Source: three-view drawing plus pictorial views. Frame: mm from the lowest corner of the part. A direction names the side the tool comes from. Coordinates: 2 decimals unless noted, no trailing zeros. Write each loop counter-clockwise with the first axis right and the second up, starting at its lowest first coordinate (ties: lowest second). Pieces come first, ordered by that corner, then holes. Notation, with made-up numbers: (-23.5, 80.25) -> (-3.5, 80.25) arc R23 cw to (-3.5, 94.25) -> close; hole circle Ø2 at (-36, 80.25). An arc over 180 degrees is marked (long way). One line per item, written item: value. Start each with the question number.
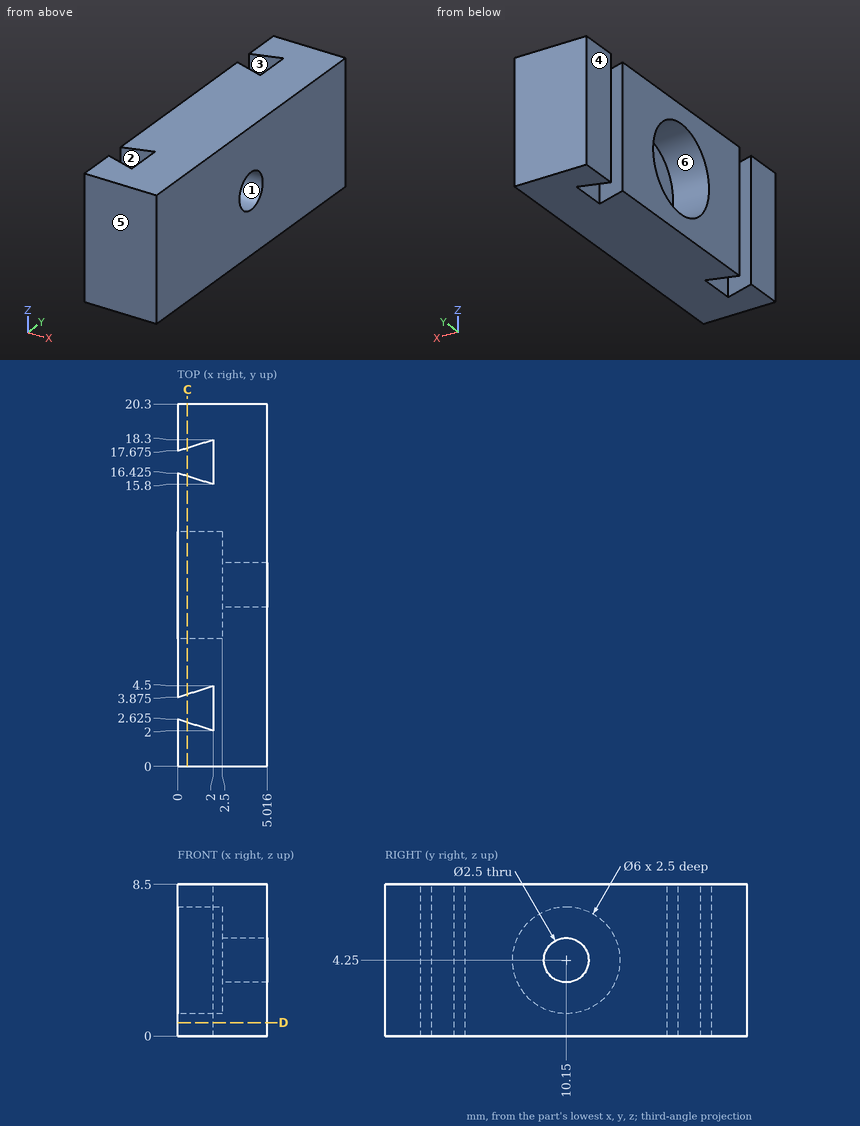
Q1. Draft query along Y for the marked faces 3, 4, 5 and 6. Return one class per face: pulls with the +Y half, pulls with the -Y half, needs draft (parallel to the pull), parting line crosses it, or undercut.
Q2. Access query for the marked faces 1 and 2. Directions: +Z, -Z, +X, -X, +Y, -Y. A direction counts if a zero-diameter tool reaches every point of the face in a straight line with its end or side. Return the directions, or none.
Q3. Line query: L1, parallel to Y at x = 3.5, z = 4.25; L2, parallel to Y at x = 1.8, z = 3; L3, parallel to Y at x = 0.9, z = 3.5 (1 decimal). Output: solid intervals per line, ascending. Write a range as from..to.
Q4. First-contact query: P1, Ø4, axis at y = 10.15, z = 4.25, coming from the -X side. Flat tip, straight axial feed; report the tip coordinate or a pass-through.
Q5. Cut plane D-D on z = 0.75. Output: boundary loops of the cut face in (x, y) (1 decimal).
Q6. Cut plane C-C on x = 0.55. Output: boundary loops of the cut face in (y, z), and give its area (3 significant figures).
Solution:
1. face 3: undercut
1. face 4: needs draft
1. face 5: pulls with the -Y half
1. face 6: undercut
2. face 1: +X, -X
2. face 2: +Z, -Z
3. L1: 0..8.9, 11.4..20.3
3. L2: 0..2.06, 4.44..7.42, 12.88..15.86, 18.24..20.3
3. L3: 0..2.3, 4.2..7.2, 13.1..16.1, 18..20.3
4. P1: x = 2.5
5. outline: (0, 0) -> (5, 0) -> (5, 20.3) -> (0, 20.3) -> (0, 17.7) -> (2, 18.3) -> (2, 15.8) -> (0, 16.4) -> (0, 3.9) -> (2, 4.5) -> (2, 2) -> (0, 2.6) -> close
6. outline: (0, 0) -> (2.45, 0) -> (2.45, 8.5) -> (0, 8.5) -> close; (4.05, 0) -> (16.25, 0) -> (16.25, 8.5) -> (4.05, 8.5) -> close; (17.85, 0) -> (20.3, 0) -> (20.3, 8.5) -> (17.85, 8.5) -> close; hole circle Ø6 at (10.15, 4.25)
6. area: 117 mm²
